```python
from build123d import *

# Parameters (mm, degrees)
SKETCH_1_R            = 18.5
EXTRUDE_312_DEPTH     = 54
SKETCH_2_R            = 8.5
CUT_EXTRUDE_18_DEPTH  = 61.004166522
SKETCH_3_R            = 11
CUT_EXTRUDE_22_DEPTH  = 35
CUT_EXTRUDE_722_DEPTH = 61.004166522
HOLE_WIZARD_M3_D      = 2.5
HOLE_WIZARD_M3_DEPTH  = 22.5
HOLE_WIZARD_M3_TIP    = 0.751075774
CUT_EXTRUDE_START     = -13
SKETCH_10_R           = 11
CUT_EXTRUDE_1_DEPTH   = 13
CHAMFER_1_SIZE        = 1


# Read off the part's stored shape, not the designer's step: Масленка M3
with BuildPart() as part:
    # Эскиз1 → Extrude 312 (new body)
    with BuildSketch(Plane(origin=(0, 0, 0), x_dir=(0, 0, -1), z_dir=(1, 0, 0))):
        Circle(SKETCH_1_R)
    extrude(amount=-EXTRUDE_312_DEPTH)

    # Эскиз2 → Вырез18 (cut, through all)
    with BuildSketch(Plane(origin=(0, 0, 0), x_dir=(0, 0, -1), z_dir=(1, 0, 0))):
        Circle(SKETCH_2_R)
    extrude(amount=-CUT_EXTRUDE_18_DEPTH, mode=Mode.SUBTRACT)

    # Эскиз3 → Вырез22 (cut)
    with BuildSketch(Plane.ZY.offset(54)):
        Circle(SKETCH_3_R)
    extrude(amount=-CUT_EXTRUDE_22_DEPTH, mode=Mode.SUBTRACT)

    # Эскиз4 → Cut-Extrude 722 (cut, through all)
    with BuildSketch(Plane(origin=(0, 0, 0), x_dir=(1, 0, 0), z_dir=(0, 1, 0))):
        with BuildLine():
            Line((-38, 3), (-32, 3))
            ThreePointArc((-32, 3), (-29, 0), (-32, -3))
            Line((-32, -3), (-38, -3))
            ThreePointArc((-38, -3), (-41, 0), (-38, 3))
        make_face()
    extrude(amount=CUT_EXTRUDE_722_DEPTH, mode=Mode.SUBTRACT)

    # Hole Wizard M3
    with Locations(Plane.ZY.offset(54)):
        with Locations((-12.773874706, 7.375), (-12.773874706, -7.375), (12.773874706, 7.375), (12.773874706, -7.375)):
            Hole(HOLE_WIZARD_M3_D / 2, depth=HOLE_WIZARD_M3_DEPTH)
            with Locations((0, 0, -(HOLE_WIZARD_M3_DEPTH + HOLE_WIZARD_M3_TIP / 2))):  # 118° drill point
                Cone(0, HOLE_WIZARD_M3_D / 2, HOLE_WIZARD_M3_TIP, mode=Mode.SUBTRACT)

    # Эскиз10 → Вырез-Вытянуть1 (cut)
    with BuildSketch(Plane(origin=(0, 0, 0), x_dir=(0, 0, -1), z_dir=(1, 0, 0)).offset(CUT_EXTRUDE_START)):
        with Locations(Location((0, 0, 0), (0, 0, 180))):
            Circle(SKETCH_10_R)
    extrude(amount=CUT_EXTRUDE_1_DEPTH, mode=Mode.SUBTRACT)

    # Фаска1
    chamfer_1_edges = [part.edges().sort_by_distance(p)[0] for p in [
        (-54, 0, -11),
        (0, 0, 18.5),
        (0, 0, -11),
    ]]
    chamfer(chamfer_1_edges, length=CHAMFER_1_SIZE)

    # Hole Wizard M3 2 outline → Hole Wizard M3 2 (revolve, cut)
    with BuildSketch(Plane(origin=(-16, 0, 0), x_dir=(1, 0, 0), z_dir=(0, 0, 1))):
        Polygon((1.12540101, 18.500010757), (1.12540101, 8.425110656), (1.250001052, 8.500000632), (1.25, 18.225), (1.25, 18.500010757), align=None)
        Polygon((0, 8.425110656), (1.125382105, 8.425110656), (1.12540101, 18.500010757), (0, 18.500010757), align=None)
        Polygon((1.25, 18.500010757), (1.25, 18.225), (1.525010757, 18.500010757), align=None)
    revolve(axis=Axis((-16, 0, 0), (0, 1, 0)), mode=Mode.SUBTRACT)


solid = part.part
```
Verification items for the finished model (mm, model axes). A direction names the side the tool comes from. Round coordinates to 2 decimals unless told otherwise and drop trailing zeros. Order: outer loops, then holes, each group sorted by start corner. A loop starts at its lowest first (then second) coordinate and runs counter-clockwise, first axis right, second up. Notation, with made-up numbers: (-37, 61) - (11, 61) arc R13 ccw to (11, 76) - close; hole circle Ø3 at (19.5, -20.5). An arc over 180 degrees is marked (long way). Use CSV: the item, a comma, the result in double quotes.
(1) Section check C-C on x = -49. Record the boundary of the cut face in (y, z) (3 decimals), and give its area (3 significant figures).
Entries:
outline,"circle Ø37 at (0, 0); hole circle Ø22 at (0, 0); hole circle Ø2.5 at (-7.375, -12.774); hole circle Ø2.5 at (-7.375, 12.774); hole circle Ø2.5 at (7.375, -12.774); hole circle Ø2.5 at (7.375, 12.774)"
area,"675 mm^2"
(2) Section check B-B on x = -16. Record the boundary of the cut face in (y, z) (3 decimals), and give its area (3 significant figures).
Entries:
outline,"(8.425, -1.125) arc R8.5 cw (long way) to (8.425, 1.125) - (8.5, 1.25) - (18.225, 1.25) - (18.442, 1.467) arc R18.5 ccw (long way) to (18.442, -1.467) - (18.225, -1.25) - (8.5, -1.25) - close"
area,"823 mm^2"
(3) Mould release check, pull along X, two halves, no side actions. Record for faces 5 (the face through (-29, 14, 0)), 6 (the face through (-42.592, 6.896, 11.619)), 7 (the face through (0, -4, 12)), 8 (the face through (-30.88, -7.19, -12.66)): released by +X, released by -X, zero draft, split by the parting line, or undercut.
Entries:
face 5,"undercut"
face 6,"zero draft"
face 7,"released by +X"
face 8,"released by -X"
(4) Gauge pin test, flat ends, axial feed: pin 1 Ø8 at (x, z) = (-13, 2) entering from -Y; pin 2 Ø1.5 at (y, z) = (7.38, 12.77) entering from -X; pin 3 Ø3 at (x, z) = (-16, 0) entering from +Y (3 decimals). Record the tip position at first contact, or that the pin passes through.
Entries:
pin 1,"y = -18.5"
pin 2,"x = -31.2"
pin 3,"y = 18.475"
(5) Access from +Z, -Z, +X, -X, +Y, -Y to the whole of each face (thin tool, end or side, straight path). Record for faces 1 (the face through (-42.592, 6.614, -11.782)), 2 (the face through (-35, 14, 3)), 3 (the face through (-15.96, -8.3, 1.84)), 4 (the face through (-13, 8.1, 3.2)).
Entries:
face 1,"-X"
face 2,"+Y"
face 3,"+X, -X"
face 4,"+X"
(6) Section check A-A on y = 0. Record the boundary of the cut face in (x, z), and give its area (3 significant figures).
Entries:
outline,"(-54, -18.5) - (-1, -18.5) - (0, -17.5) - (0, -12) - (-1, -11) - (-13, -11) - (-13, -8.5) - (-19, -8.5) - (-19, -11) - (-53, -11) - (-54, -12) - close; (-54, 12) - (-53, 11) - (-19, 11) - (-19, 8.5) - (-13, 8.5) - (-13, 11) - (-1, 11) - (0, 12) - (0, 17.5) - (-1, 18.5) - (-54, 18.5) - close"
area,"837 mm^2"
(7) Thickness scan on probe 1 along Y at (x, z) = (-5.25, 0); probe 2 along Z at (x, y) = (-9, 3); probe 3 along Z at (x, y) = (-30, 16.5). Record the ranges inside material, lowest first. Write a range as from..to.
Entries:
probe 1,"-18.5..-11, 11..18.5"
probe 2,"-18.26..-10.58, 10.58..18.26"
probe 3,"-8.37..-2.24, 2.24..8.37"
